Work out the finished part from the listing and answer in its coordinate system (mm). Face numbers are marked on the shaded views. A direction names the side the tool comes from. Coordinates: 2 decimals unless noted, no trailing zeros. Order: outer loops, then holes, each group sorted by start corner. A loop starts at its lowest first (then second) coordinate and runs counter-clockwise, first axis right, second up. Notation, with made-up numbers: M 85.5,-25 L 114.5,-25 A16 ccw 114.5,-6 Z; hole C 6,23.5 d1. An arc over 180 degrees is marked long. Use a Markdown table: item, result.
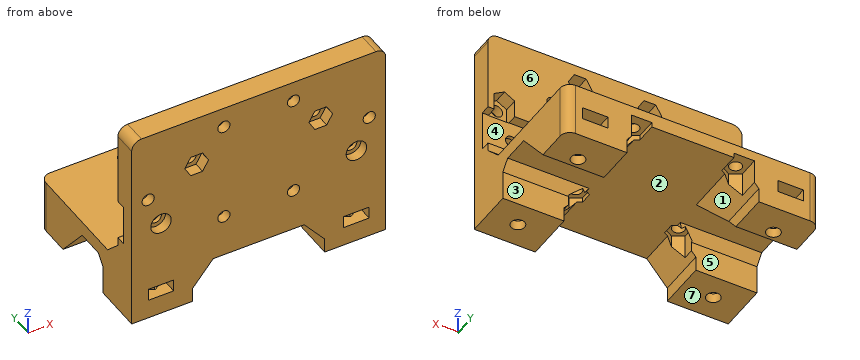
from build123d import *

# Parameters (mm, degrees)
PAD009_DEPTH         = 26
SKETCH025_R          = 1.25
POCKET011_DEPTH      = 32.001
POCKET012_DEPTH      = 32.001
SKETCH031_R          = 1.4
POCKET015_DEPTH      = 9
POCKET016_DEPTH      = 2
POCKET017_DEPTH      = 2.5
SKETCH034_R          = 1.25
POCKET018_DEPTH      = 41.501
SKETCH035_R          = 3
POCKET019_DEPTH      = 30.501
POCKET020_DEPTH      = 9.001
POCKET021_DEPTH      = 30.001
POCKET022_DEPTH      = 32.001
POCKET023_DEPTH      = 41.501
SKETCH046_R          = 1.25
POCKET026_DEPTH      = 32.001
POCKET027_DEPTH      = 2.3
POCKET034_DEPTH      = 26.001
POCKET034_DEPTH_BACK = 26.001
SKETCH065_W          = 52.3
SKETCH065_H          = 8.3
POCKET035_DEPTH      = 29.201
SKETCH066_R          = 1.25
POCKET036_DEPTH      = 32.001
SKETCH067_R          = 2.1
POCKET037_DEPTH      = 2


with BuildPart() as part:
    # Sketch016 → Pad009 (new body, symmetric)
    with BuildSketch(Plane.YZ):
        Polygon((0, 0), (32, 0), (32, 11), (8.4, 11), (4.8, 14.6), (4.8, 41.5), (0, 41.5), align=None)
    extrude(amount=PAD009_DEPTH, both=True)

    # Sketch025 → Pocket011 (cut, through all)
    with BuildSketch(Plane.XZ):
        with Locations((-22.625, 27)):
            Circle(SKETCH025_R)
        with Locations((7.125, 37.25)):
            Circle(SKETCH025_R)
        with Locations((7.125, 16.75)):
            Circle(SKETCH025_R)
        with Locations((-7.125, 37.25)):
            Circle(SKETCH025_R)
        with Locations((-7.125, 16.75)):
            Circle(SKETCH025_R)
        with Locations((22.625, 27)):
            Circle(SKETCH025_R)
    extrude(amount=-POCKET011_DEPTH, mode=Mode.SUBTRACT)

    # Sketch026 → Pocket012 (cut, through all)
    with BuildSketch(Plane.XZ):
        Polygon((-13.5, 0), (13.5, 0), (13.5, 3), (9.304502, 8), (-9.304502, 8), (-13.5, 3), align=None)
    extrude(amount=-POCKET012_DEPTH, mode=Mode.SUBTRACT)

    # Sketch031 → Pocket015 (cut)
    with BuildSketch(Plane.XY):
        with Locations((-20, 26)):
            Circle(SKETCH031_R)
        with Locations((20, 26)):
            Circle(SKETCH031_R)
        with Locations((-20, 5)):
            Circle(SKETCH031_R)
        with Locations((20, 5)):
            Circle(SKETCH031_R)
    extrude(amount=POCKET015_DEPTH, mode=Mode.SUBTRACT)

    # Sketch032 (on DatumPlane) → Pocket016 (cut)
    with BuildSketch(Plane.XY.offset(2)):
        Polygon((-20, 29.002221), (-22.6, 27.501111), (-22.6, 24.498889), (-20, 22.997779), (-17.4, 24.498889), (-17.4, 27.501111), align=None)
        Polygon((20, 29.002221), (17.4, 27.501111), (17.4, 24.498889), (20, 22.997779), (22.6, 24.498889), (22.6, 27.501111), align=None)
        Polygon((-20, 8.002221), (-22.6, 6.501111), (-22.6, 3.498889), (-20, 1.997779), (-17.4, 3.498889), (-17.4, 6.501111), align=None)
        Polygon((20, 8.002221), (17.4, 6.501111), (17.4, 3.498889), (20, 1.997779), (22.6, 3.498889), (22.6, 6.501111), align=None)
    extrude(amount=POCKET016_DEPTH, mode=Mode.SUBTRACT)

    # Sketch033 (on DatumPlane) → Pocket017 (cut)
    with BuildSketch(Plane.XY.offset(4)):
        Polygon((-20, 22.997779), (-17.4, 24.498889), (-17.4, 27.501111), (-17.4, 47.501111), (-22.6, 47.501111), (-22.6, 27.501111), (-22.6, 24.498889), align=None)
        Polygon((20, 22.997779), (22.6, 24.498889), (22.6, 27.501111), (22.6, 47.501111), (17.4, 47.501111), (17.4, 27.501111), (17.4, 24.498889), align=None)
        Polygon((-20, 8.002221), (-22.6, 6.501111), (-22.6, 3.498889), (-22.6, -16.501111), (-17.4, -16.501111), (-17.4, 3.498889), (-17.4, 6.501111), align=None)
        Polygon((20, 8.002221), (17.4, 6.501111), (17.4, 3.498889), (17.4, -16.501111), (22.6, -16.501111), (22.6, 3.498889), (22.6, 6.501111), align=None)
    extrude(amount=POCKET017_DEPTH, mode=Mode.SUBTRACT)

    # Sketch034 → Pocket018 (cut, through all)
    with BuildSketch(Plane.XY):
        with Locations((-10.5, 29)):
            Circle(SKETCH034_R)
        with Locations((10.5, 29)):
            Circle(SKETCH034_R)
        with Locations((10.5, 9)):
            Circle(SKETCH034_R)
        with Locations((-10.5, 9)):
            Circle(SKETCH034_R)
    extrude(amount=POCKET018_DEPTH, mode=Mode.SUBTRACT)

    # Sketch035 (on DatumPlane) → Pocket019 (cut, through all)
    with BuildSketch(Plane.XY.offset(11)):
        with Locations((-10.5, 9)):
            Circle(SKETCH035_R)
        with Locations((10.5, 9)):
            Circle(SKETCH035_R)
    extrude(amount=POCKET019_DEPTH, mode=Mode.SUBTRACT)

    # Sketch036 (on DatumPlane) → Pocket020 (cut, through all)
    with BuildSketch(Plane.XY.offset(9)):
        Polygon((-10.5, 26.575129), (-8.4, 27.787564), (-8.4, 30.212436), (-8.4, 46.212436), (-12.6, 46.212436), (-12.6, 30.212436), (-12.6, 27.787564), align=None)
        Polygon((10.5, 26.575129), (12.6, 27.787564), (12.6, 30.212436), (12.6, 46.212436), (8.4, 46.212436), (8.4, 30.212436), (8.4, 27.787564), align=None)
        Polygon((-10.5, 11.424871), (-12.6, 10.212436), (-12.6, 7.787564), (-10.5, 6.575129), (-8.4, 7.787564), (-8.4, 10.212436), align=None)
        Polygon((10.5, 11.424871), (8.4, 10.212436), (8.4, 7.787564), (10.5, 6.575129), (12.6, 7.787564), (12.6, 10.212436), align=None)
    extrude(amount=-POCKET020_DEPTH, mode=Mode.SUBTRACT)

    # Sketch037 (on DatumPlane) → Pocket021 (cut, through all)
    with BuildSketch(Plane.XZ.offset(-2)):
        Polygon((-22.625, 29.424871), (-24.725, 28.212436), (-24.725, 25.787564), (-24.725, 24.575129), (-20.525, 24.575129), (-20.525, 25.787564), (-20.525, 28.212436), align=None)
        Polygon((4.700129, 37.25), (5.912564, 35.15), (8.337436, 35.15), (9.549871, 37.25), (8.337436, 39.35), (5.912564, 39.35), align=None)
        Polygon((4.700129, 16.75), (5.912564, 14.65), (8.337436, 14.65), (9.549871, 16.75), (8.337436, 18.85), (5.912564, 18.85), align=None)
        Polygon((-4.700129, 37.25), (-5.912564, 39.35), (-8.337436, 39.35), (-9.549871, 37.25), (-8.337436, 35.15), (-5.912564, 35.15), align=None)
        Polygon((-9.549871, 16.75), (-8.337436, 14.65), (-5.912564, 14.65), (-4.700129, 16.75), (-5.912564, 18.85), (-8.337436, 18.85), align=None)
        Polygon((22.625, 29.424871), (20.525, 28.212436), (20.525, 25.787564), (20.525, 24.575129), (24.725, 24.575129), (24.725, 25.787564), (24.725, 28.212436), align=None)
    extrude(amount=-POCKET021_DEPTH, mode=Mode.SUBTRACT)

    # Sketch038 → Pocket022 (cut, through all)
    with BuildSketch(Plane.XZ):
        with BuildLine():
            Line((-24, 41.5), (24, 41.5))
            ThreePointArc((26, 39.5), (25.414214, 40.914214), (24, 41.5))
            Line((26, 39.5), (26, 0))
            Line((26, 0), (36, 0))
            Line((36, 51.5), (36, 0))
            Line((-36, 51.5), (36, 51.5))
            Line((-36, 0), (-36, 51.5))
            Line((-26, 0), (-36, 0))
            Line((-26, 39.5), (-26, 0))
            ThreePointArc((-24, 41.5), (-25.414214, 40.914214), (-26, 39.5))
        make_face()
    extrude(amount=-POCKET022_DEPTH, mode=Mode.SUBTRACT)

    # Sketch039 → Pocket023 (cut, through all)
    with BuildSketch(Plane.XY):
        with BuildLine():
            Line((-26, 0), (-26, 30))
            ThreePointArc((-24, 32), (-25.414214, 31.414214), (-26, 30))
            Line((-24, 32), (24, 32))
            ThreePointArc((26, 30), (25.414214, 31.414214), (24, 32))
            Line((26, 30), (26, 0))
            Line((26, 0), (36, 0))
            Line((36, 42), (36, 0))
            Line((-36, 42), (36, 42))
            Line((-36, 0), (-36, 42))
            Line((-26, 0), (-36, 0))
        make_face()
    extrude(amount=POCKET023_DEPTH, mode=Mode.SUBTRACT)

    # Sketch046 → Pocket026 (cut, through all)
    with BuildSketch(Plane.XZ):
        with Locations((-12.7, 31)):
            Circle(SKETCH046_R)
        with Locations((12.7, 31)):
            Circle(SKETCH046_R)
    extrude(amount=-POCKET026_DEPTH, mode=Mode.SUBTRACT)

    # Sketch047 → Pocket027 (cut)
    with BuildSketch(Plane.XZ):
        Polygon((15.124871, 31), (13.912436, 33.1), (11.487564, 33.1), (10.275129, 31), (11.487564, 28.9), (13.912436, 28.9), align=None)
        Polygon((-10.275129, 31), (-11.487564, 33.1), (-13.912436, 33.1), (-15.124871, 31), (-13.912436, 28.9), (-11.487564, 28.9), align=None)
    extrude(amount=-POCKET027_DEPTH, mode=Mode.SUBTRACT)

    # Sketch064 → Pocket034 (cut, two sides)
    with BuildSketch(Plane.YZ) as pocket034_sk:
        Polygon((10, 0), (24, 0), (17.287203, 8), (11.678199, 8), (10, 6), align=None)
    extrude(amount=-POCKET034_DEPTH, mode=Mode.SUBTRACT)
    extrude(pocket034_sk.sketch, amount=POCKET034_DEPTH_BACK, mode=Mode.SUBTRACT)

    # Sketch065 (on DatumPlane) → Pocket035 (cut, through all)
    with BuildSketch(Plane.XZ.offset(-2.8)):
        with Locations((0, 20.5)):
            Rectangle(SKETCH065_W, SKETCH065_H)
    extrude(amount=-POCKET035_DEPTH, mode=Mode.SUBTRACT)

    # Sketch066 → Pocket036 (cut, through all)
    with BuildSketch(Plane.XZ):
        with Locations((-20, 20.5)):
            Circle(SKETCH066_R)
        with Locations((20, 20.5)):
            Circle(SKETCH066_R)
    extrude(amount=-POCKET036_DEPTH, mode=Mode.SUBTRACT)

    # Sketch067 → Pocket037 (cut)
    with BuildSketch(Plane.XZ):
        with Locations((-20, 20.5)):
            Circle(SKETCH067_R)
        with Locations((20, 20.5)):
            Circle(SKETCH067_R)
    extrude(amount=-POCKET037_DEPTH, mode=Mode.SUBTRACT)


solid = part.part
1. Section C-C on y = 19.5 is taken. Determine the outline of the cut face in (x, z), then the cut area to 3 significant figures.
Answers below:
| item | result |
|---|---|
| outline | M -26,5.36 L -11.52,5.36 L -9.3,8 L 9.3,8 L 11.52,5.36 L 26,5.36 L 26,11 L -26,11 Z |
| area | 238 mm² |
2. For the marked faces 1, 2, 3 and 4, determine the directions among +Z, -Z, +X, -X, +Y, -Y from which every point of the face is accessible in a straight line to the end or side of a thin tool.
Answers below:
| item | result |
|---|---|
| face 1 | -Z, +Y, -Y |
| face 2 | -Z |
| face 3 | -Z, +X, -X |
| face 4 | +X, -X, +Y |
3. Section B-B on z = 34 is taken. Determine the outline of the cut face in (x, y), then the cut area to 3 significant figures.
Answers below:
| item | result |
|---|---|
| outline | M -26,0 L 26,0 L 26,4.8 L -26,4.8 Z |
| area | 250 mm² |
4. Flat-ended cylindrical pins translate along their axes: P1, Ø1.3, axis at x = 12.5, z = 32, coming from the -Y side; P2, Ø1.3, axis at x = -19, y = 30, coming from the +Z side; P3, Ø3, axis at x = 7.5, y = 5, coming from the -Z side. Find the tip coordinate at first contact, or state that the pin passes through.
Answers below:
| item | result |
|---|---|
| P1 | y = 2.3 |
| P2 | z = 11 |
| P3 | z = 8 |
5. Find the intervals of material crossed by probe 1 along X at (y, z) = (9, 10.35); probe 2 along X at (y, z) = (26, 0.55); probe 3 along Y at (x, z) = (20, 7.4), in increasing order.
Answers below:
| item | result |
|---|---|
| probe 1 | -26 to -11.75, -9.25 to 9.25, 11.75 to 26 |
| probe 2 | -26 to -21.4, -18.6 to -13.5, 13.5 to 18.6, 21.4 to 26 |
| probe 3 | 0 to 3.6, 6.4 to 11.17, 17.79 to 24.6, 27.4 to 32 |
6. Section D-D on x = 16.5 is taken. Determine the outline of the cut face in (y, z).
Answers below:
| item | result |
|---|---|
| outline | M 0,0 L 10,0 L 10,6 L 11.68,8 L 17.29,8 L 24,0 L 32,0 L 32,11 L 8.4,11 L 4.8,14.6 L 4.8,16.35 L 2.8,16.35 L 2.8,24.65 L 4.8,24.65 L 4.8,41.5 L 0,41.5 Z |
7. For a pull along Y with two mould halves and no side action, classify the marked faces 5, 6 and 7 as +Y half, -Y half, draft (parallel to the pull), parting line (faces both ways), or undercut.
Answers below:
| item | result |
|---|---|
| face 5 | undercut |
| face 6 | +Y half |
| face 7 | draft |
8. Section A-A on x = 2.5 is taken. Determine the outline of the cut face in (y, z), then the cut area to 3 significant figures.
Answers below:
| item | result |
|---|---|
| outline | M 0,8 L 32,8 L 32,11 L 8.4,11 L 4.8,14.6 L 4.8,16.35 L 2.8,16.35 L 2.8,24.65 L 4.8,24.65 L 4.8,41.5 L 0,41.5 Z |
| area | 232 mm² |
